Print and shaded views of the part. All mm, measured from the part's lowest x, y and z. A direction names the side the tool comes from. Coordinates: 2 decimals unless noted, no trailing zeros. Loops run counter-clockwise (first coordinate to the right, second up) from the corner with the lowest first, then second, coordinate; pieces in that order, holes last.
1) Pin check, flat tips, straight feed: pin 1 Ø2 at (y, z) = (8.5, 8) entering from -X; pin 2 Ø4 at (x, z) = (8.5, 7.5) entering from +Y; pin 3 Ø3 at (x, z) = (5, 4.815) entering from +Y; pin 4 Ø3.5 at (x, y) = (11, 7) entering from +Z. Stop position of each tip, or through.
2) Saw through at C-C, the plane z = 2. Write the cut outline in (x, y).
3) Wall check: line 1 along X through (y, z) = (7.25, 3.25); line 2 along Z through (x, y) = (17, 5) (3 decimals); line 3 along Y through (x, z) = (11.5, 2.25). Give the ranges that are in metal, low to high.
4) Saw through at B-B, the plane y = 7.5. Give the number of separate pieces and of enclosed holes in the cut face, and give its area (3 significant figures).
5) Saw through at D-D, the plane y = 1. Write the cut outline in (x, z) (3 decimals), and give its area (3 significant figures).
6) Which spindle directions (+Z, -Z, +X, -X, +Y, -Y) get a long thin tool onto all of the face, cutting with end or side? Do the marked faces 4 and 5. Say none if no direction does.
7) Saw through at A-A, the plane x = 11. Write the cut outline in (y, z).
8) Two-plate mould, pull along Z, no slides. Class the marked faces 1, 2 and 3: +Z half, -Z half, draft (parallel to the pull), parting line (faces both ways), or undercut.
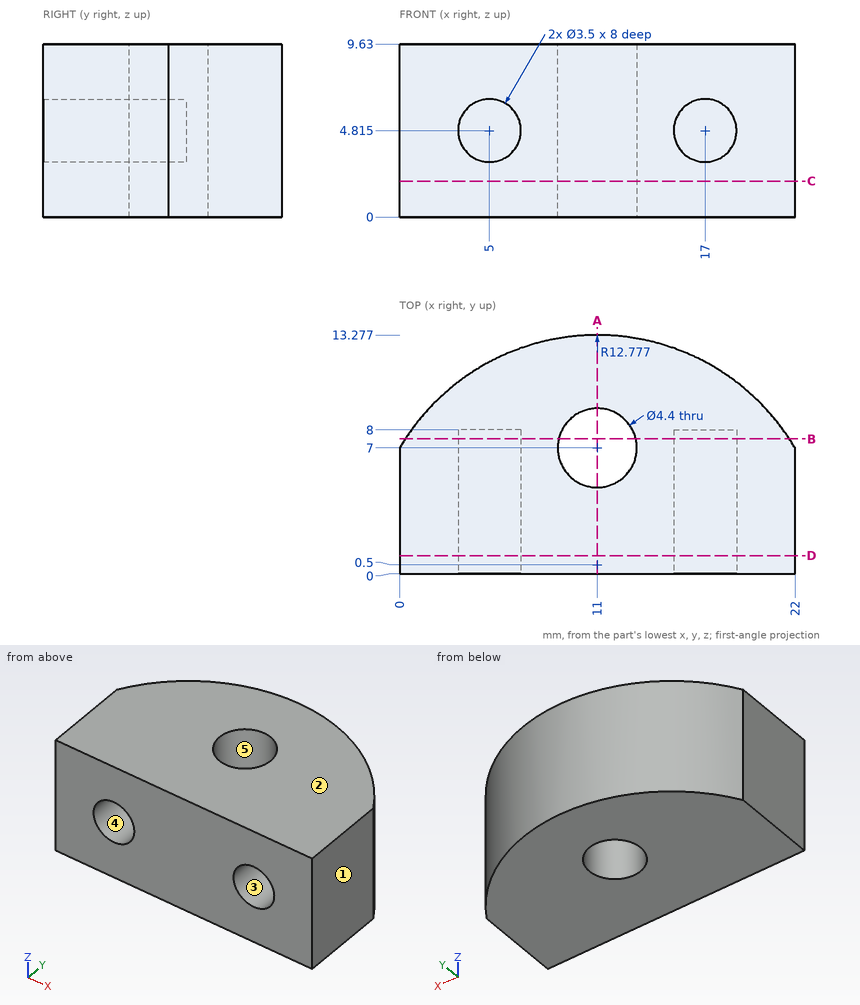
Data:
1. pin 1: stops at x = 0.31
1. pin 2: stops at y = 13.27
1. pin 3: stops at y = 12.46
1. pin 4: passes through
2. outline: (0, 0) - (22, 0) - (22, 7) arc R12.78 ccw to (0, 7) - close; hole circle Ø4.4 at (11, 7)
3. line 1: x = 0.15 to 4.22, 5.78 to 8.81, 13.19 to 16.22, 17.78 to 21.85
3. line 2: z = 0 to 3.065, 6.565 to 9.63
3. line 3: y = 0 to 4.86, 9.14 to 13.27
4. separate pieces: 2
4. enclosed holes: 2
4. area: 145 mm2
5. outline: (0, 0) - (22, 0) - (22, 9.63) - (0, 9.63) - close; hole circle Ø3.5 at (5, 4.815); hole circle Ø3.5 at (17, 4.815)
5. area: 193 mm2
6. face 4: -Y
6. face 5: +Z, -Z
7. outline: (0, 0) - (4.8, 0) - (4.8, 9.63) - (0, 9.63) - close; (9.2, 0) - (13.28, 0) - (13.28, 9.63) - (9.2, 9.63) - close
8. face 1: draft
8. face 2: +Z half
8. face 3: undercut
